```python
from build123d import *
from build123d.topology import SkipClean

# Parameters (mm, degrees)
EXTRUDE_1_DEPTH          = 80
SKETCH_2_R               = 13
CUT_EXTRUDE_2_DEPTH      = 15
CUT_EXTRUDE_START        = -15
SKETCH_4_R               = 13
CUT_EXTRUDE_3_DEPTH      = 15
CUT_EXTRUDE_4_DEPTH      = 123.918354375
CUT_EXTRUDE_4_DEPTH_BACK = 123.918354375
SKETCH_5_W               = 20
SKETCH_5_H               = 40
CUT_EXTRUDE_6_DEPTH      = 123.918354375
CUT_EXTRUDE_6_DEPTH_BACK = 24
CUT_EXTRUDE_7_DEPTH      = 131.345394404
CUT_EXTRUDE_8_DEPTH      = 32
CUT_EXTRUDE_8_DEPTH_BACK = 24
SKETCH_10_W              = 30
SKETCH_10_H              = 40
CUT_EXTRUDE_9_DEPTH      = 6
SKETCH_13_W              = 10.619852086
SKETCH_13_H              = 40
CUT_EXTRUDE_10_DEPTH     = 71
EXTRUDE_3_DEPTH          = 60
FILLET_1_R               = 3
SKETCH_14_R              = 25
CUT_EXTRUDE_11_DEPTH     = 50
CUT_EXTRUDE_START_2      = -95
SKETCH_16_R              = 13
CUT_EXTRUDE_12_DEPTH     = 95
SKETCH_17_W              = 10
SKETCH_17_H              = 50
EXTRUDE_4_DEPTH          = 16
SKETCH_20_W              = 10
SKETCH_20_H              = 50
EXTRUDE_5_DEPTH          = 20


with BuildPart() as part:
    # Эскиз1 → Бобышка-Вытянуть1 (new body)
    with BuildSketch(Plane.XY):
        with BuildLine():
            Line((-84.314422505, -30), (-23.694570419, 25.759800711))
            ThreePointArc((-23.694570419, 25.759800711), (28.113366731, 20.847988178), (17.769230769, -30.153846154))
            Line((17.769230769, -30.153846154), (1.060606061, -40))
            Line((1.060606061, -40), (-84.314422505, -40))
            Line((-84.314422505, -40), (-84.314422505, -30))
        make_face()
    extrude(amount=EXTRUDE_1_DEPTH)

    # Эскиз2 → Вырез-Вытянуть2 (cut)
    with BuildSketch(Plane.XY):
        Circle(SKETCH_2_R)
    extrude(amount=CUT_EXTRUDE_2_DEPTH, mode=Mode.SUBTRACT)

    # Эскиз4 → Вырез-Вытянуть3 (cut)
    with BuildSketch(Plane.XY.offset(80).offset(CUT_EXTRUDE_START)):
        Circle(SKETCH_4_R)
    extrude(amount=CUT_EXTRUDE_3_DEPTH, mode=Mode.SUBTRACT)

    # Эскиз5 → Вырез-Вытянуть4 (cut, two sides: drawn at the far end of the back side and taken through both)
    with BuildSketch(Plane(origin=(0, 0, 0), x_dir=(1, 0, 0), z_dir=(0, 1, 0)).offset(-CUT_EXTRUDE_4_DEPTH_BACK)):
        with Locations((-74.314422505, -40)):
            Rectangle(SKETCH_5_W, SKETCH_5_H)
    extrude(amount=CUT_EXTRUDE_4_DEPTH + CUT_EXTRUDE_4_DEPTH_BACK, mode=Mode.SUBTRACT)

    # Эскиз6 → Вырез-Вытянуть6 (cut, two sides: drawn at the far end of the back side and taken through both)
    with BuildSketch(Plane(origin=(0, 0, 0), x_dir=(1, 0, 0), z_dir=(0, 1, 0)).offset(-CUT_EXTRUDE_6_DEPTH_BACK)):
        with BuildLine():
            Line((-55, -25), (-84.314422505, -25))
            Line((-84.314422505, -25), (-84.314422505, -55))
            Line((-84.314422505, -55), (-55, -55))
            ThreePointArc((-55, -55), (-40, -40), (-55, -25))
        make_face()
    extrude(amount=CUT_EXTRUDE_6_DEPTH + CUT_EXTRUDE_6_DEPTH_BACK, mode=Mode.SUBTRACT)

    # Эскиз9 → Вырез-Вытянуть7 (cut, through all)
    with BuildSketch(Plane(origin=(0, -24, 0), x_dir=(1, 0, 0), z_dir=(0, 1, 0))):
        with BuildLine():
            Line((-55, -48), (-92.733432528, -48))
            Line((-92.733432528, -48), (-92.733432528, -32))
            Line((-92.733432528, -32), (-55, -32))
            ThreePointArc((-55, -32), (-47, -40), (-55, -48))
        make_face()
    extrude(amount=-CUT_EXTRUDE_7_DEPTH, mode=Mode.SUBTRACT)

    # Эскиз10 → Вырез-Вытянуть8 (cut, two sides: drawn at the far end of the back side and taken through both)
    with BuildSketch(Plane(origin=(0, 0, 0), x_dir=(1, 0, 0), z_dir=(0, 1, 0)).offset(-CUT_EXTRUDE_8_DEPTH_BACK)):
        with Locations((-49.314422505, -40)):
            Rectangle(SKETCH_10_W, SKETCH_10_H)
    extrude(amount=CUT_EXTRUDE_8_DEPTH + CUT_EXTRUDE_8_DEPTH_BACK, mode=Mode.SUBTRACT)

    # Эскиз11 → Вырез-Вытянуть9 (cut)
    with BuildSketch(Plane(origin=(0, -24, 0), x_dir=(1, 0, 0), z_dir=(0, 1, 0))):
        with BuildLine():
            Line((-55, -25), (-81.861005174, -25))
            Line((-81.861005174, -25), (-81.861005174, -55))
            Line((-81.861005174, -55), (-55, -55))
            ThreePointArc((-55, -55), (-40, -40), (-55, -25))
        make_face()
    extrude(amount=-CUT_EXTRUDE_9_DEPTH, mode=Mode.SUBTRACT)

    # Эскиз13 → Вырез-Вытянуть10 (cut)
    with BuildSketch(Plane(origin=(0, -24, 0), x_dir=(1, 0, 0), z_dir=(0, 1, 0))):
        with Locations((-29.004496462, -40)):
            Rectangle(SKETCH_13_W, SKETCH_13_H)
    extrude(amount=CUT_EXTRUDE_10_DEPTH, mode=Mode.SUBTRACT)

    # Эскиз12 → Бобышка-Вытянуть3 (add)
    with SkipClean():  # the faces are left unmerged after this step: merging them gives an invalid solid
        with BuildSketch(Plane.XY):
            with BuildLine():
                Line((-35, 0), (-35, -24))
                Line((-35, -24), (-25.475478406, -24))
                ThreePointArc((-25.475478406, -24), (32.53184397, 12.9104271), (-35, 0))
            make_face()
        extrude(amount=EXTRUDE_3_DEPTH)

    # Скругление1
    fillet_1_edges = [part.edges().sort_by_distance(p)[0] for p in [
        (-35, -24, 40),
    ]]
    fillet(fillet_1_edges, radius=FILLET_1_R)

    # Эскиз14 → Вырез-Вытянуть11 (cut)
    with SkipClean():  # the faces are left unmerged after this step: merging them gives an invalid solid
        with BuildSketch(Plane.XY.offset(65)):
            Circle(SKETCH_14_R)
        extrude(amount=-CUT_EXTRUDE_11_DEPTH, mode=Mode.SUBTRACT)

    # Эскиз16 → Вырез-Вытянуть12 (cut)
    with SkipClean():  # the faces are left unmerged after this step: merging them gives an invalid solid
        with BuildSketch(Plane.XY.offset(80).offset(CUT_EXTRUDE_START_2)):
            Circle(SKETCH_16_R)
        extrude(amount=CUT_EXTRUDE_12_DEPTH, mode=Mode.SUBTRACT)

    # Эскиз17 → Бобышка-Вытянуть4 (add)
    with SkipClean():  # the faces are left unmerged after this step: merging them gives an invalid solid
        with BuildSketch(Plane(origin=(0, 15, 0), x_dir=(1, 0, 0), z_dir=(0, 1, 0))):
            with Locations((0.685577495, -40)):
                Rectangle(SKETCH_17_W, SKETCH_17_H)
        extrude(amount=EXTRUDE_4_DEPTH)

    # Эскиз20 → Бобышка-Вытянуть5 (add)
    with SkipClean():  # the faces are left unmerged after this step: merging them gives an invalid solid
        with BuildSketch(Plane(origin=(0, -15, 0), x_dir=(1, 0, 0), z_dir=(0, 1, 0))):
            with Locations((0.685577495, -40)):
                Rectangle(SKETCH_20_W, SKETCH_20_H)
        extrude(amount=-EXTRUDE_5_DEPTH)


solid = part.part
```
Could you check a few things on this model? Use its own coordinates, in mm. A direction names the side the tool comes from. Give positions to 0.01 mm unless a question says otherwise; leave off trailing zeros. Order: outer loops, then holes, each group sorted by start corner. A loop starts at its lowest first (then second) coordinate and runs counter-clockwise, first axis right, second up.
Q1. Suppose I cut it at D-D, the plane y = -10. Write out the boundary of the cut face in (x, z), and give its area (3 significant figures).
Q2. Suppose I cut it at B-B, the plane x = -66. Write out the boundary of the cut face in (y, z).
Q3. For faces 4 (the flat face through (-56, -15, 60)), 5 (the flat face through (-60, -35, 32)), 6 (the flat face through (1, 15, 40)), 7 (the cylindrical face through (-10.316, -7.91, 7.395)), which set-ups out of +Z, -Z, +X, -X, +Y, -Y let a thin tool reach every point of the face, with its end or its side?
Q4. If I drill on line 1 along Y through (x, z) = (0, 6); line 2 along Z through (x, y) = (9.5, 14); line 3 along X through (y, z) = (-17, 63), over which ranges is the centre line in solid material (lowest first)?
Q5. I'm going to push flat-ended pins straight in: P1, Ø5, axis at y = -4.5, z = 25.5, coming from the +X side; P2, Ø3, axis at y = -21, z = 47, coming from the +X side; P3, Ø13, axis at x = -57.5, z = 45.5, coming from the +Y side. Where does each tip first touch, or does it pass through?
Q6. Suppose I cut it at A-A, the plane z = 40. Write out the boundary of the cut face in (x, y), and give its area (3 significant figures).
Q7. We'd pull the mould along X, two halves only. Please class faces 1 (the flat face through (-54.43, -2.51, 9.86)), 2 (the cylindrical face through (-10.316, -7.91, 72.395)), 3 (the flat face through (-60, -35, 48)): +X half, -X half, draft (parallel to the pull), parting line (faces both ways), or undercut.
Q8. Suppose I cut it at C-C, the plane y = 19.5. Write out the boundary of the cut face in (x, z), and give its area (3 significant figures).
Solution:
1. outline: (-62.57, 0) - (-8.31, 0) - (-8.31, 15) - (-22.91, 15) - (-22.91, 65) - (-8.31, 65) - (-8.31, 80) - (-62.57, 80) - (-62.57, 60) - (-35, 60) - (-35, 20) - (-62.57, 20) - close; (8.31, 0) - (33.54, 0) - (33.54, 80) - (8.31, 80) - (8.31, 65) - (22.91, 65) - (22.91, 15) - (8.31, 15) - close
1. area: 3,800 mm2
2. outline: (-40, 0) - (-13.15, 0) - (-13.15, 20) - (-40, 20) - close; (-40, 60) - (-13.15, 60) - (-13.15, 80) - (-40, 80) - close
3. face 4: -X, +Y
3. face 5: -X, +Y, -Y
3. face 6: none
3. face 7: +Z, -Z
4. line 1: y = -40 to -13, 13 to 35
4. line 2: z = 0 to 15, 65 to 80
4. line 3: x = -70.18 to -18.33, -4.31 to 5.69, 18.33 to 30.59
5. P1: stops at x = 34.94
5. P2: stops at x = 29.06
5. P3: stops at y = -30
6. outline: (-47, -40) - (1.06, -40) - (17.77, -30.15) arc R35 ccw (long way) to (-35, 0) - (-35, -21) arc R3 cw to (-38, -24) - (-40, -24) - (-40, -30) - (-47, -30) - close; hole (-4.31, -24.62) - (-4.31, -15) - (5.69, -15) - (5.69, -24.34) arc R25 ccw to (5.69, 24.34) - (5.69, 15) - (-4.31, 15) - (-4.31, 24.62) arc R25 ccw to start
6. area: 2,710 mm2
7. face 1: -X half
7. face 2: undercut
7. face 3: draft
8. outline: (-30.5, 0) - (29.06, 0) - (29.06, 80) - (-30.5, 80) - (-30.5, 60) - (-29.06, 60) - (-29.06, 20) - (-30.5, 20) - close; hole (-15.64, 15) - (-4.31, 15) - (-4.31, 65) - (-15.64, 65) - close; hole (5.69, 15) - (15.64, 15) - (15.64, 65) - (5.69, 65) - close
8. area: 3,640 mm2
